The model under review builds one solid part; all positions refer to its coordinate system, in mm. A direction names the side the tool comes from. Give positions to 0.01 mm unless a question says otherwise; leave off trailing zeros. Order: outer loops, then holes, each group sorted by start corner. A loop starts at its lowest first (then second) coordinate and runs counter-clockwise, first axis right, second up. Notation, with made-up numbers: (85, 35) - (131, 35) arc R31 ccw to (131, 67) - close; hole circle Ø10 at (26.5, 32.25). An arc over 180 degrees is marked (long way). Use CSV: the item, a comma, the result in double quotes.
```python
from build123d import *

# Parameters (mm, degrees)
SKETCH2_R          = 1.5
CUT_EXTRUDE1_DEPTH = 5


with BuildPart() as part:
    # Sketch1 → Revolve1 (revolve)
    with BuildSketch(Plane.XY):
        Polygon((0, 0), (100.4, 0), (100.4, 16), (19.3, 16), (19.3, 9), (15.5, 9), (15.5, 3), (0, 3), align=None)
    revolve(axis=Axis((0, 0, 0), (1, 0, 0)))

    # Sketch2 → Cut-Extrude1 (cut)
    with BuildSketch(Plane.ZY.offset(-19.3)):
        with Locations((0, 13)):
            Circle(SKETCH2_R)
        with Locations((0, -13)):
            Circle(SKETCH2_R)
        with Locations((-13, 0)):
            Circle(SKETCH2_R)
        with Locations((13, 0)):
            Circle(SKETCH2_R)
    extrude(amount=-CUT_EXTRUDE1_DEPTH, mode=Mode.SUBTRACT)


solid = part.part
```
Item 1: Tool access review of faces 1 (the face through (100.4, 0, 0)), 2 (the face through (24.3, 0, 13)): name each direction out of +Z, -Z, +X, -X, +Y, -Y from which nothing blocks a thin tool from reaching the whole face with its end or side.
Results list:
face 1,"+Z, -Z, +X, +Y, -Y"
face 2,"-X"
Item 2: Take a section at C-C, the plane z = 7. Give the boundary of the cut face in (x, y), and give its area (3 significant figures).
Results list:
outline,"(15.5, -5.66) - (19.3, -5.66) - (19.3, -14.39) - (100.4, -14.39) - (100.4, 14.39) - (19.3, 14.39) - (19.3, 5.66) - (15.5, 5.66) - close"
area,"2,380 mm2"
Item 3: Take a section at A-A, the plane y = 0. Give the boundary of the cut face in (x, z).
Results list:
outline,"(0, -3) - (15.5, -3) - (15.5, -9) - (19.3, -9) - (19.3, -11.5) - (24.3, -11.5) - (24.3, -14.5) - (19.3, -14.5) - (19.3, -16) - (100.4, -16) - (100.4, 16) - (19.3, 16) - (19.3, 14.5) - (24.3, 14.5) - (24.3, 11.5) - (19.3, 11.5) - (19.3, 9) - (15.5, 9) - (15.5, 3) - (0, 3) - close"
Item 4: Take a section at D-D, the plane x = 65. Give the boundary of the cut face in (y, z).
Results list:
outline,"circle Ø32 at (0, 0)"
Item 5: Clearance check with flat-ended pins moving along their axes: pin 1 (1 mm diameter, centred on y = 3.5, z = -5, fed in from -X); pin 2 (2 mm diameter, centred on x = 56.5, z = -3.5, fed in from -Y); pin 3 (5 mm diameter, centred on x = 15, y = -6.5, fed in from +Z). State where each tip first meets the part, or that it passes through.
Results list:
pin 1,"stops at x = 15.5"
pin 2,"stops at y = -15.8"
pin 3,"stops at z = 8.04"
Item 6: Mouldability with a two-part tool opening along Z and no side actions: class faces 3 (the face through (17.373, -1.172, 8.923)), 4 (the face through (24.3, -13, 0)), 5 (the face through (0, 0, 0)) as pulls with the +Z half, pulls with the -Z half, needs draft (parallel to the pull), parting line crosses it, or undercut.
Results list:
face 3,"parting line crosses it"
face 4,"undercut"
face 5,"needs draft"
Item 7: Wall thickness on L1, parallel to X at y = -2, z = -2.5; L2, parallel to X at y = 11, z = 5; L3, parallel to Y at x = 20, z = -13: over which ranges is each line inside the solid? List them lowest first.
Results list:
L1,"x = 15.5 to 100.4"
L2,"x = 19.3 to 100.4"
L3,"y = -9.33 to -1.5, 1.5 to 9.33"
Item 8: Take a section at B-B, the plane x = 22. Give the boundary of the cut face in (y, z), and give its area (3 significant figures).
Results list:
outline,"circle Ø32 at (0, 0); hole circle Ø3 at (-13, 0); hole circle Ø3 at (0, -13); hole circle Ø3 at (0, 13); hole circle Ø3 at (13, 0)"
area,"776 mm2"
